Can you work these out from the model? Positions are in its coordinate system, mm. A direction names the side the tool comes from. Give positions to 0.01 mm unless a question says otherwise; leave off trailing zeros. Loops run counter-clockwise (first coordinate to the right, second up) from the corner with the lowest first, then second, coordinate; pieces in that order, holes last. Notation, with made-up numbers: (87.5, 23) - (99.5, 23) arc R13 cw to (99.5, 30) - close; hole circle Ø5 at (34, 82.5). An arc over 180 degrees is marked (long way). Answer as a JSON object with one key per item and string values.
```python
from build123d import *

# Parameters (mm, degrees)
SKETCH1_R                = 5
SKETCH1_R_2              = 1
BOSS_EXTRUDE1_DEPTH      = 10
BOSS_EXTRUDE2_DEPTH      = 40
BOSS_EXTRUDE2_DEPTH_BACK = 10
SKETCH2_W                = 8
SKETCH2_H                = 5
BOSS_EXTRUDE3_DEPTH      = 40
BOSS_EXTRUDE3_DEPTH_BACK = 8
SKETCH3_W                = 10
SKETCH3_H                = 5


with BuildPart() as part:
    # Sketch1 → Boss-Extrude1 (new body)
    with BuildSketch(Plane.XY):
        with BuildLine():
            Line((-9.16515139, 2.5), (-100, 2.5))
            Line((-100, 2.5), (-100, -2.5))
            Line((-100, -2.5), (-9.16515139, -2.5))
            ThreePointArc((-9.16515139, -2.5), (9.5, 0), (-9.16515139, 2.5))
        make_face()
        Circle(SKETCH1_R, mode=Mode.SUBTRACT)
        with Locations((2.755362887, -7)):
            Circle(SKETCH1_R_2, mode=Mode.SUBTRACT)
        with Locations((-3.001411686, -6.89808325)):
            Circle(SKETCH1_R_2, mode=Mode.SUBTRACT)
        with Locations((-7, -2.755362887)):
            Circle(SKETCH1_R_2, mode=Mode.SUBTRACT)
        with Locations((-6.89808325, 3.001411686)):
            Circle(SKETCH1_R_2, mode=Mode.SUBTRACT)
        with Locations((-2.755362887, 7)):
            Circle(SKETCH1_R_2, mode=Mode.SUBTRACT)
        with Locations((3.001411686, 6.89808325)):
            Circle(SKETCH1_R_2, mode=Mode.SUBTRACT)
        with Locations((7, 2.755362887)):
            Circle(SKETCH1_R_2, mode=Mode.SUBTRACT)
        with Locations((6.89808325, -3.001411686)):
            Circle(SKETCH1_R_2, mode=Mode.SUBTRACT)
    extrude(amount=BOSS_EXTRUDE1_DEPTH)

    # Sketch2 → Boss-Extrude2 (add, two sides: drawn at the far end of the back side and taken through both)
    with BuildSketch(Plane.XY.offset(10).offset(-BOSS_EXTRUDE2_DEPTH_BACK)):
        with Locations((-104, 0)):
            Rectangle(SKETCH2_W, SKETCH2_H)
    extrude(amount=BOSS_EXTRUDE2_DEPTH + BOSS_EXTRUDE2_DEPTH_BACK)

    # Sketch3 → Boss-Extrude3 (add, two sides: drawn at the far end of the back side and taken through both)
    with BuildSketch(Plane.ZY.offset(108).offset(-BOSS_EXTRUDE3_DEPTH_BACK)):
        with Locations((55, 0)):
            Rectangle(SKETCH3_W, SKETCH3_H)
    extrude(amount=BOSS_EXTRUDE3_DEPTH + BOSS_EXTRUDE3_DEPTH_BACK)


solid = part.part
```
1) If we mould it in two halves opening along Y, with no side actions, what happens to faces 1 (the flat face through (-83, -2.5, 8)), 2 (the flat face through (-83, 2.5, 8)), 3 (the cylindrical face through (-1.08, -4.88, 4.93))? For each: released by +Y, released by -Y, zero draft, split by the parting line, or undercut.
Check sheet entries:
{"face 1": "released by -Y", "face 2": "released by +Y", "face 3": "undercut"}
2) Imagine slicing it at D-D on x = -106.5. Write out the boundary of the cut face in (y, z).
Check sheet entries:
{"outline": "(-2.5, 0) - (2.5, 0) - (2.5, 60) - (-2.5, 60) - close"}
3) Imagine slicing it at B-B on y = 0. Write out the boundary of the cut face in (x, z).
Check sheet entries:
{"outline": "(-148, 50) - (-108, 50) - (-108, 0) - (-5, 0) - (-5, 10) - (-100, 10) - (-100, 60) - (-148, 60) - close; (5, 0) - (9.5, 0) - (9.5, 10) - (5, 10) - close"}
4) I need wall thicknesses on L1, parallel to X at y = -7.5, z = 7; L2, parallel to X at y = -0.5, z = 7; L3, parallel to Z at x = -76, y = 2. Which ranges of each line are inside material? Lowest first, please.
Check sheet entries:
{"L1": "-5.83 to -3.8, -2.2 to 1.89, 3.62 to 5.83", "L2": "-108 to -4.97, 4.97 to 9.49", "L3": "0 to 10"}
5) Imagine slicing it at C-C on z = 37.5. Write out the boundary of the cut face in (x, y), and give its area (3 significant figures).
Check sheet entries:
{"outline": "(-108, -2.5) - (-100, -2.5) - (-100, 2.5) - (-108, 2.5) - close", "area": "40.0 mm2"}
6) Which directions (+Z, -Z, +X, -X, +Y, -Y) give clear straight access to the entire face, cutting with the end or side of a thin tool? Please do faces 4 (the flat face through (-148, 0, 55)), 5 (the flat face through (-100, 0, 35)), 6 (the flat face through (-108, 0, 25)).
Check sheet entries:
{"face 4": "+Z, -Z, -X, +Y, -Y", "face 5": "+Z, +X, +Y, -Y", "face 6": "-Z, -X, +Y, -Y"}
7) Imagine slicing it at A-A on x = 0. Write out the boundary of the cut face in (y, z).
Check sheet entries:
{"outline": "(-9.5, 0) - (-5, 0) - (-5, 10) - (-9.5, 10) - close; (5, 0) - (9.5, 0) - (9.5, 10) - (5, 10) - close"}
8) I'm going to push flat-ended pins straight in: P1, Ø1.5, axis at y = 1, z = 12.5, coming from the -X side; P2, Ø5, axis at x = -42, y = 2.5, coming from the +Z side; P3, Ø3, axis at y = -3.5, z = 36, coming from the +X side. Where does each tip first touch, or does it pass through?
Check sheet entries:
{"P1": "x = -108", "P2": "z = 10", "P3": "x = -100"}
